The figure shows three views and two pictorial views of one solid part (mm, origin at its lowest corner). Answer the questions. Coordinates: 2 decimals unless noted, no trailing zeros. Loops run counter-clockwise (first coordinate to the right, second up) from the corner with the lowest first, then second, coordinate; pieces in that order, holes last. Notation, with made-up numbers: M 59.5,-0.75 L 91.5,-0.75 A28 cw 91.5,18.25 Z; hole C 5,-26.5 d3. An arc over 180 degrees is marked long. Answer in a Markdown table with one row per item. Add a question column.
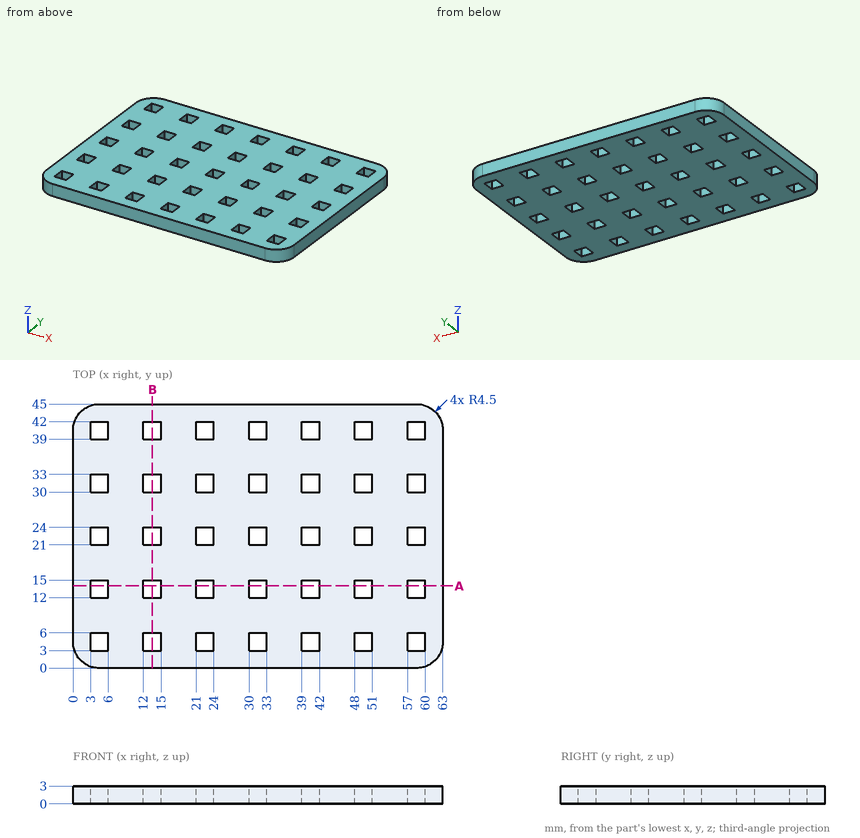
(1) A cutting plane is placed at A-A (y = 14). State how many separate pieces and enclosed holes the cut face has, plus the area to 3 significant figures.
(2) A cutting plane is placed at B-B (x = 13.5). Give the vertices of the cut face in (y, z), plus the area to 3 significant figures.
(3) Straight lines are drawn through the part: line 1 (Y direction, x = 22.5, z = 1.05); line 2 (Y direction, x = 3.5, z = 2.75). For each, find the intervals that lie inside material, in ascending order.
Solved:
| question | item | result |
|---|---|---|
| 1 | separate pieces | 8 |
| 1 | enclosed holes | 0 |
| 1 | area | 126 mm² |
| 2 | outline | M 0,0 L 3,0 L 3,3 L 0,3 Z; M 6,0 L 12,0 L 12,3 L 6,3 Z; M 15,0 L 21,0 L 21,3 L 15,3 Z; M 24,0 L 30,0 L 30,3 L 24,3 Z; M 33,0 L 39,0 L 39,3 L 33,3 Z; M 42,0 L 45,0 L 45,3 L 42,3 Z |
| 2 | area | 90.0 mm² |
| 3 | line 1 | y = 0 to 3, 6 to 12, 15 to 21, 24 to 30, 33 to 39, 42 to 45 |
| 3 | line 2 | y = 0.11 to 3, 6 to 12, 15 to 21, 24 to 30, 33 to 39, 42 to 44.89 |
